The drawing under review shows one solid part. Ordinate dimensions are in mm from its lowest x, y, z. A direction names the side the tool comes from. Give positions to 0.01 mm unless a question says otherwise; leave off trailing zeros. Write each loop counter-clockwise with the first axis right and the second up, starting at its lowest first coordinate (ties: lowest second). Pieces come first, ordered by that corner, then holes. Notation, with made-up numbers: M 4.5,11.5 L 23.5,11.5 A22 cw 23.5,35.5 Z; hole C 34,-39 d1. An arc over 180 degrees is marked long. Use one line per item in the form item = value. Start each with the question number.
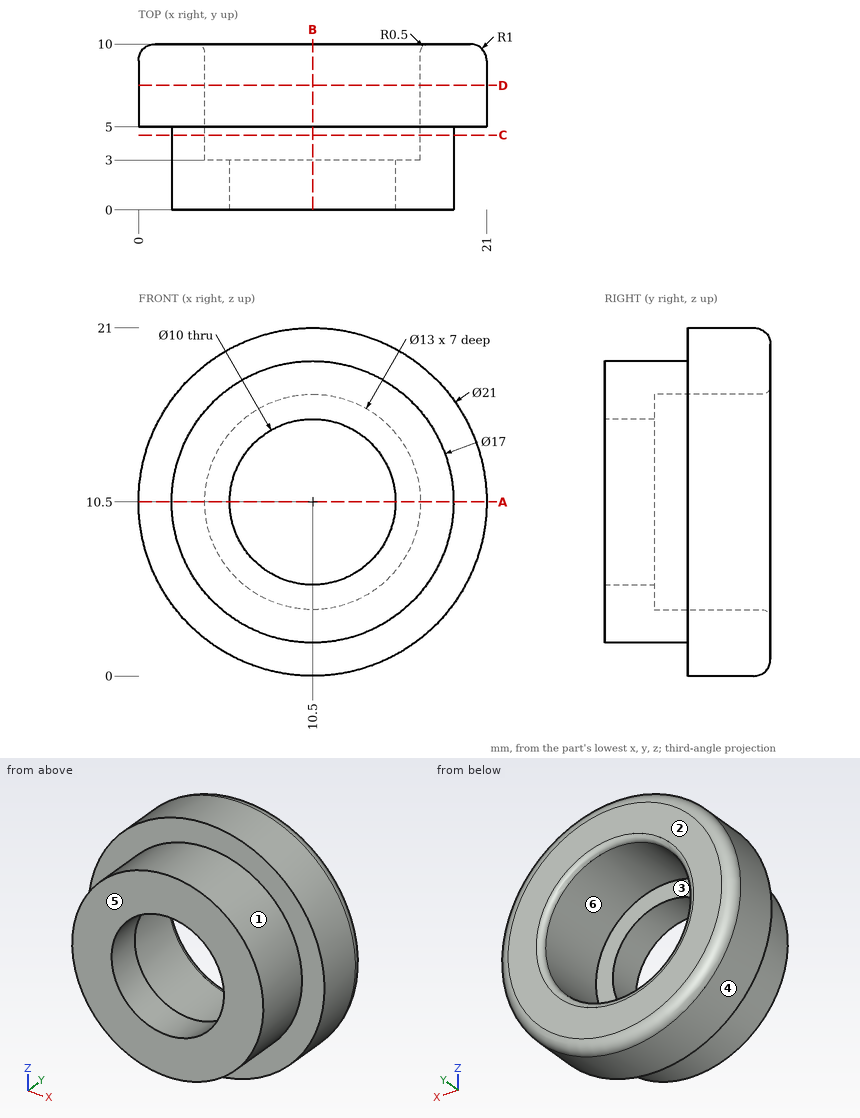
1. Draft analysis for pull direction X (two halves, no side actions). For the marked faces 3, 4, 5 and 6, state which applies: pulls with the +X half, pulls with the -X half, needs draft (parallel to the pull), parting line crosses it, or undercut.
2. Clearance check with flat-ended pins moving along their axes: pin 1 Ø2 at (x, y) = (14, 8.5) entering from +Z; pin 2 Ø4 at (y, z) = (3.5, 4.5) entering from +X; pin 3 Ø1.5 at (y, z) = (2.5, 7.5) entering from +X; pin 4 Ø8 at (x, z) = (10.5, 10.5) entering from -Y. State where each tip first meets the part, or that it passes through.
3. We need section D-D (y = 7.5). State the section outline as (x, z) points, and give its area (3 significant figures).
4. To check wall thickness, follow L1, parallel to X at y = 7.75, z = 10.5; L2, parallel to X at y = 1.45, z = 10.5; L3, parallel to Y at x = 15.25, z = 14.25. State the ranges of each line that lie inside material, in increasing order.
5. We need section A-A (z = 10.5). State the section outline as (x, y) points.
6. For the marked faces 1 and 2, list the 3-axis set-ups (+Z, -Z, +X, -X, +Y, -Y) from which the entire face can be reached by the end or side of a thin tool; tool diameter is ignored.
7. We need section B-B (x = 10.5). State the section outline as (y, z) points, and give its area (3 significant figures).
8. We need section C-C (y = 4.5). State the section outline as (x, z) points.
Answer block:
q1.face_3 = undercut
q1.face_4 = parting line crosses it
q1.face_5 = needs draft
q1.face_6 = undercut
q2.pin_1 = 20.7
q2.pin_2 = 19.9
q2.pin_3 = 18.7
q2.pin_4 = through
q3.outline = C 10.5,10.5 d21; hole C 10.5,10.5 d13
q3.area = 214 mm^2
q4.L1 = 0 to 4, 17 to 21
q4.L2 = 2 to 5.5, 15.5 to 19
q4.L3 = 0 to 3
q5.outline = M 0,5 L 2,5 L 2,0 L 5.5,0 L 5.5,3 L 4,3 L 4,9.5 A0.5 ccw 3.5,10 L 1,10 A1 ccw 0,9 Z; M 15.5,0 L 19,0 L 19,5 L 21,5 L 21,9 A1 ccw 20,10 L 17.5,10 A0.5 ccw 17,9.5 L 17,3 L 15.5,3 Z
q6.face_1 = -Y
q6.face_2 = +Z, -Z, +X, -X, +Y
q7.outline = M 0,2 L 5,2 L 5,0 L 9,0 A1 ccw 10,1 L 10,3.5 A0.5 ccw 9.5,4 L 3,4 L 3,5.5 L 0,5.5 Z; M 0,15.5 L 3,15.5 L 3,17 L 9.5,17 A0.5 ccw 10,17.5 L 10,20 A1 ccw 9,21 L 5,21 L 5,19 L 0,19 Z
q7.area = 68.5 mm^2
q8.outline = C 10.5,10.5 d17; hole C 10.5,10.5 d13
